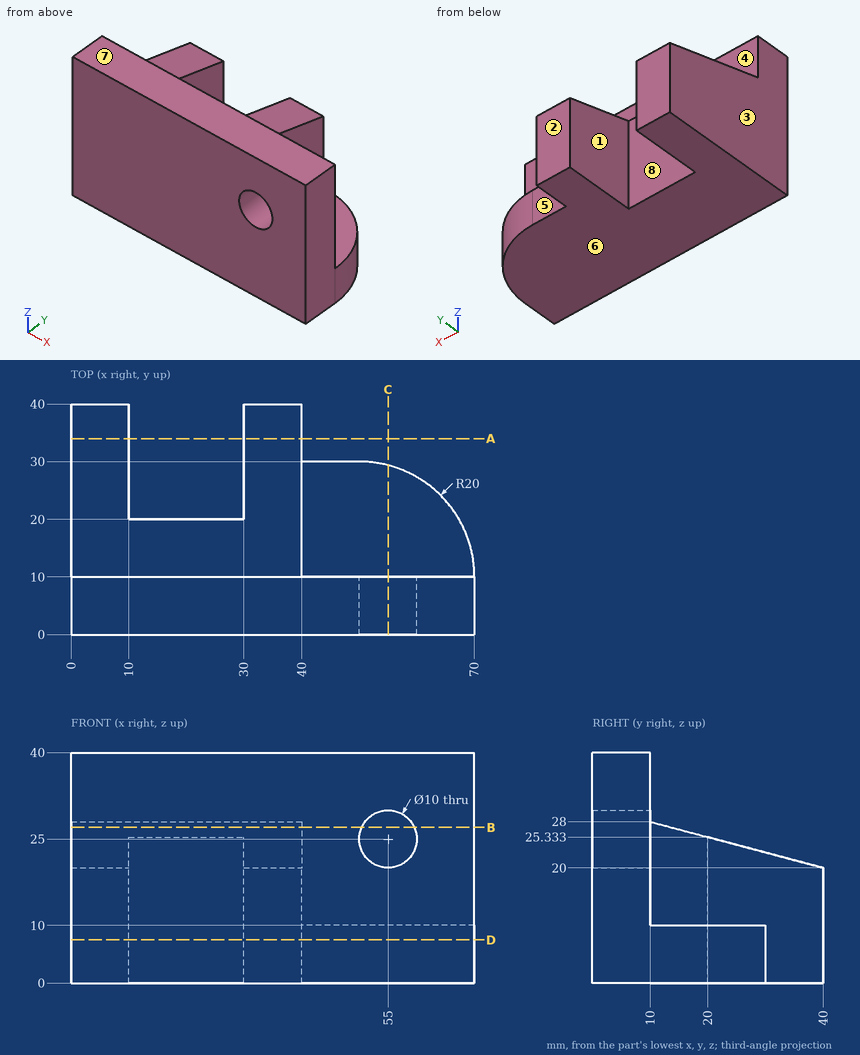
Answer from the drawing. Dimensions are ordinates in mm from the lowest x, y and z of the part. A direction names the side the tool comes from. Give positions to 0.01 mm unless a question says otherwise; leave off trailing zeros. Order: outer loops, then holes, each group sorted by start corner. A loop starts at its lowest first (then second) coordinate and runs counter-clockwise, first axis right, second up. Notation, with made-up numbers: (85, 67) - (111, 67) arc R20 cw to (111, 71) - close; hole circle Ø11 at (67.5, 37.25). An arc over 180 degrees is marked (long way). One line per item, written item: value. Start each with the question number.
1) A cutting plane is placed at D-D on z = 7.5. Give the vertices of the cut face in (x, y).
2) Find the intervals of material crossed by L1, parallel to X at y = 29, z = 13.5; L2, parallel to Z at x = 55, y = 5.5; L3, parallel to X at y = 3.25, z = 25, in increasing order.
3) Given pin 1 Ø22 at (y, z) = (25.5, 7.5) entering from +X; pin 2 Ø11 at (x, z) = (46.5, 6.5) entering from +Y; pin 3 Ø1 at (y, z) = (23, 13) entering from +X, each flat-ended and moving along its own axis, determine where each tip first touches the part or whether it passes through.
4) A cutting plane is placed at C-C on x = 55. Give the vertices of the cut face in (y, z) (1 decimal).
5) A cutting plane is placed at A-A on y = 34. Give the vertices of the cut face in (x, z), then the cut area to 3 significant figures.
6) A cutting plane is placed at B-B on z = 27. Give the vertices of the cut face in (x, y).
7) A tool of negligible diameter and unlimited length cuts with its end or side. For the marked faces 4, 5, 6, 7 and 8, from which of +Z, -Z, +X, -X, +Y, -Y can it reach the whole face along a straight path? Write none if from no direction.
8) The mould has two halves that part along X. Classify the marked faces 1, 2 and 3: released by +X, released by -X, zero draft, split by the parting line, or undercut.
Answer sheet:
1. outline: (0, 0) - (70, 0) - (70, 10) arc R20 ccw to (50, 30) - (40, 30) - (40, 40) - (30, 40) - (30, 20) - (10, 20) - (10, 40) - (0, 40) - close
2. L1: x = 0 to 10, 30 to 40
2. L2: z = 0 to 20, 30 to 40
2. L3: x = 0 to 50, 60 to 70
3. pin 1: stops at x = 69.49
3. pin 2: stops at y = 30
3. pin 3: stops at x = 40
4. outline: (0, 0) - (29.4, 0) - (29.4, 10) - (10, 10) - (10, 20) - (0, 20) - close; (0, 30) - (10, 30) - (10, 40) - (0, 40) - close
5. outline: (0, 0) - (10, 0) - (10, 21.6) - (0, 21.6) - close; (30, 0) - (40, 0) - (40, 21.6) - (30, 21.6) - close
5. area: 432 mm2
6. outline: (0, 0) - (50.42, 0) - (50.42, 10) - (40, 10) - (40, 13.75) - (0, 13.75) - close; (59.58, 0) - (70, 0) - (70, 10) - (59.58, 10) - close
7. face 4: +Z, +X, +Y
7. face 5: +Z, -Z, +X, +Y
7. face 6: -Z, +X, -X, +Y, -Y
7. face 7: +Z, +X, -X, +Y, -Y
7. face 8: +Z, -Z, +Y
8. face 1: undercut
8. face 2: zero draft
8. face 3: released by -X
